```python
from build123d import *

# Parameters (mm, degrees)
SKETCH_W        = 91.1
SKETCH_H        = 44.5
PAD_DEPTH       = 3.55
SKETCH001_R     = 6.1
SKETCH001_W     = 31.8
SKETCH001_H     = 12.2
SKETCH001_W_2   = 23.5
SKETCH001_H_2   = 2
SKETCH001_W_3   = 20
SKETCH001_H_3   = 5
POCKET_DEPTH    = 7.101
SKETCH002_R     = 1.6
SKETCH002_R_2   = 1.55
POCKET001_DEPTH = 42.501
POCKET002_DEPTH = 5.5
POCKET003_DEPTH = 5.5
SKETCH006_R     = 1.4
POCKET004_DEPTH = 15


with BuildPart() as part:
    # Sketch → Pad (new body, symmetric)
    with BuildSketch(Plane.XY):
        with Locations((45.55, 0)):
            Rectangle(SKETCH_W, SKETCH_H)
    extrude(amount=PAD_DEPTH, both=True)

    # Sketch001 → Pocket (cut, through all)
    with BuildSketch(Plane.XY.offset(3.55)):
        with Locations((38, 3)):
            Circle(SKETCH001_R)
        with Locations((20, 0)):
            Circle(SKETCH001_R)
        Polygon((91.1, 22.25), (91.1, 11.85), (53.1, 11.85), (5.4, 22.25), align=None)
        Polygon((91.1, -22.25), (91.1, -9.45), (66.1, -9.45), (53.1, -22.25), align=None)
        with Locations((72.75, 1.15)):
            Rectangle(SKETCH001_W, SKETCH001_H)
        with Locations((11.75, -21.25)):
            Rectangle(SKETCH001_W_2, SKETCH001_H_2)
        with Locations((39.6, -16.85)):
            Rectangle(SKETCH001_W_3, SKETCH001_H_3)
    extrude(amount=-POCKET_DEPTH, mode=Mode.SUBTRACT)

    # Sketch002 → Pocket001 (cut, through all)
    with BuildSketch(Plane.XZ.offset(20.25)):
        with Locations((3.55, 0)):
            Circle(SKETCH002_R)
        with Locations((84, 0)):
            Circle(SKETCH002_R_2)
        with BuildLine():
            Line((-1.450012, 3.55), (3.549988, 3.55))
            ThreePointArc((3.549988, 3.55), (0, 0), (3.549988, -3.55))
            Line((3.549988, -3.55), (-1.450012, -3.55))
            Line((-1.450012, -3.55), (-1.450012, 3.55))
        make_face()
    extrude(amount=-POCKET001_DEPTH, mode=Mode.SUBTRACT)

    # Sketch004 → Pocket002 (cut)
    with BuildSketch(Plane.XZ.offset(20.25)):
        with BuildLine():
            Line((0, 3.55), (23.5, 3.55))
            Line((23.5, 3.55), (23.5, 2.55))
            Line((23.5, 2.55), (3.55, 2.55))
            ThreePointArc((3.55, 2.55), (1, 0), (3.55, -2.55))
            Line((3.55, -2.55), (23.5, -2.55))
            Line((23.5, -2.55), (23.5, -3.55))
            Line((23.5, -3.55), (0, -3.55))
            Line((0, -3.55), (0, 3.55))
        make_face()
    extrude(amount=-POCKET002_DEPTH, mode=Mode.SUBTRACT)

    # Sketch005 → Pocket003 (cut)
    with BuildSketch(Plane(origin=(0, 22.25, 0), x_dir=(-1, 0, 0), z_dir=(0, 1, 0))):
        with BuildLine():
            Line((-53.1, 3.55), (0, 3.55))
            Line((0, 3.55), (0, -3.55))
            Line((0, -3.55), (-53.1, -3.55))
            Line((-53.1, -2.55), (-53.1, -3.55))
            Line((-3.55, -2.55), (-53.1, -2.55))
            ThreePointArc((-3.55, -2.55), (-1, 0), (-3.55, 2.55))
            Line((-53.1, 2.55), (-3.55, 2.55))
            Line((-53.1, 3.55), (-53.1, 2.55))
        make_face()
    extrude(amount=-POCKET003_DEPTH, mode=Mode.SUBTRACT)

    # Sketch006 → Pocket004 (cut)
    with BuildSketch(Plane.XZ.offset(22.25)):
        with Locations((37.3, 0)):
            Circle(SKETCH006_R)
        with Locations((41.8, 0)):
            Circle(SKETCH006_R)
    extrude(amount=-POCKET004_DEPTH, mode=Mode.SUBTRACT)


solid = part.part
```
Geometry check sheet. Reference: the model listing, model coordinates, mm. A direction names the side the tool comes from. Coordinates: 2 decimals unless noted, no trailing zeros. Order: outer loops, then holes, each group sorted by start corner. A loop starts at its lowest first (then second) coordinate and runs counter-clockwise, first axis right, second up.
Item 1: Section check C-C (x = 37.3). Enter the section's corners in (y, z), plus the area to 3 significant figures.
Item 2: Section check D-D (y = -12). Enter the section's corners in (x, z).
Item 3: Tool access check on faces 1 (the cylindrical face through (38.635, -20.82, 0.421)), 2 (the cylindrical face through (1, -18, 0)), 3 (the flat face through (14, -18, 2.55)), 4 (the flat face through (14, 19, -2.55)). Record the directions out of +Z, -Z, +X, -X, +Y, -Y that give a thin tool (end or side, any length) a straight path to the whole face; none if there is none.
Item 4: Depth check by flat-ended pin: pin 1 (2.5 mm diameter, centred on y = -15.5, z = -1, fed in from +X) (3 decimals); pin 2 (1.4 mm diameter, centred on x = 37.5, z = 0, fed in from -Y); pin 3 (1.5 mm diameter, centred on x = 32.5, z = 0, fed in from +Y). Enter the tip coordinate at first touch or a pass-through.
Item 5: Section check B-B (y = 3). Enter the section's corners in (x, z).
Item 6: Section check A-A (x = 76). Enter the section's corners in (y, z).
Item 7: Scan lines: line 1 along Y through (x, z) = (80, -2.75); line 2 along Z through (x, y) = (41.8, -21.6). Record each from-to range of solid material in increasing order.
Item 8: Mould release check, pull along Y, two halves, no side actions. Record for faces 5 (the flat face through (56.85, 1, 0)), 6 (the flat face through (79, -9.45, 0)), 7 (the flat face through (72, 11.85, 0)), 8 (the cylindrical face through (40.4, -20.82, 0.06)): released by +Y, released by -Y, zero draft, split by the parting line, or undercut.
Check sheet entries:
1. outline: (-22.25, -3.55) - (-19.35, -3.55) - (-19.35, -1.4) - (-22.25, -1.4) - close; (-22.25, 1.4) - (-19.35, 1.4) - (-19.35, 3.55) - (-22.25, 3.55) - close; (-14.35, -3.55) - (-3.06, -3.55) - (-3.06, 3.55) - (-14.35, 3.55) - (-14.35, 1.4) - (-7.25, 1.4) - (-7.25, -1.4) - (-14.35, -1.4) - close; (9.06, -3.55) - (15.29, -3.55) - (15.29, 3.55) - (9.06, 3.55) - close
1. area: 117 mm2
2. outline: (3.55, -3.55) - (63.51, -3.55) - (63.51, 3.55) - (3.55, 3.55) arc R3.55 ccw to start; hole circle Ø3.2 at (3.55, 0); hole circle Ø2.8 at (37.3, 0); hole circle Ø2.8 at (41.8, 0)
3. face 1: -Y
3. face 2: -X, -Y
3. face 3: +Z, -X, -Y
3. face 4: -Z, +X, -X, +Y
4. pin 1: stops at x = 61.225
4. pin 2: stops at y = -7.25
4. pin 3: stops at y = 16.5
5. outline: (3.55, -3.55) - (14.69, -3.55) - (14.69, 3.55) - (3.55, 3.55) arc R3.55 ccw to start; (25.31, -3.55) - (31.9, -3.55) - (31.9, 3.55) - (25.31, 3.55) - close; (44.1, -3.55) - (56.85, -3.55) - (56.85, 3.55) - (44.1, 3.55) - close; (88.65, -3.55) - (91.1, -3.55) - (91.1, 3.55) - (88.65, 3.55) - close; hole circle Ø3.2 at (3.55, 0)
6. outline: (-9.45, -3.55) - (-4.95, -3.55) - (-4.95, 3.55) - (-9.45, 3.55) - close; (7.25, -3.55) - (11.85, -3.55) - (11.85, 3.55) - (7.25, 3.55) - close
7. line 1: y = -9.45 to -4.95, 7.25 to 11.85
7. line 2: z = -3.55 to -1.4, 1.4 to 3.55
8. face 5: undercut
8. face 6: released by -Y
8. face 7: released by +Y
8. face 8: zero draft
